Can you work these out from the drawing? Everything is in mm from the part's minimum corner. Coordinates: 2 decimals unless noted, no trailing zeros. Loops run counter-clockwise (first coordinate to the right, second up) from the corner with the lowest first, then second, coordinate; pieces in that order, holes last. Notation, with made-up numbers: (11, 87.25) - (32, 87.25) arc R21 ccw to (32, 102.25) - close; hole circle Ø10 at (51.5, 36). An arc over 180 degrees is marked (long way). Use CSV: the item, a comma, the result in double quotes.
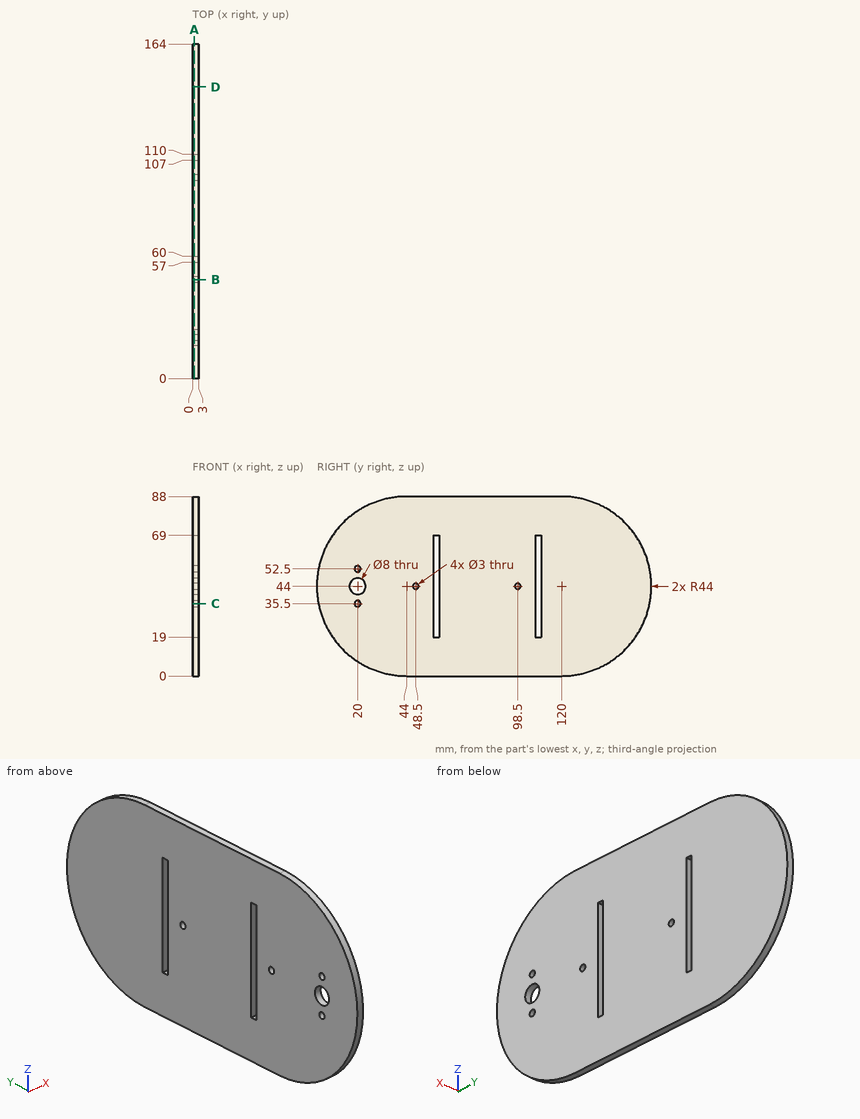
(1) Suppose I cut it at A-A (x = 0.8). Write out the boundary of the cut face in (y, z).
Computed:
outline,"(44, 0) - (120, 0) arc R44 ccw to (120, 88) - (44, 88) arc R44 ccw to start; hole circle Ø8 at (20, 44); hole circle Ø3 at (20, 35.5); hole circle Ø3 at (20, 52.5); hole circle Ø3 at (48.5, 44); hole (57, 19) - (60, 19) - (60, 69) - (57, 69) - close; hole circle Ø3 at (98.5, 44); hole (107, 19) - (110, 19) - (110, 69) - (107, 69) - close"
(2) Suppose I cut it at D-D (y = 143). Write out the boundary of the cut face in (x, z), plus the area to 3 significant figures.
Computed:
outline,"(0, 6.49) - (3, 6.49) - (3, 81.51) - (0, 81.51) - close"
area,"225 mm²"
(3) Please list where these lines run through material, in increasing order: line 1 (Y direction, x = 1.9, z = 44); line 2 (Y direction, x = 0.7, z = 67); line 3 (Y direction, x = 0.6, z = 35.5).
Computed:
line 1,"y = 0 to 16, 24 to 47, 50 to 57, 60 to 97, 100 to 107, 110 to 164"
line 2,"y = 6.49 to 57, 60 to 107, 110 to 157.51"
line 3,"y = 0.83 to 18.5, 21.5 to 57, 60 to 107, 110 to 163.17"
(4) Suppose I cut it at C-C (z = 35.5). Write out the boundary of the cut face in (x, y), plus the area to 3 significant figures.
Computed:
outline,"(0, 0.83) - (3, 0.83) - (3, 18.5) - (0, 18.5) - close; (0, 21.5) - (3, 21.5) - (3, 57) - (0, 57) - close; (0, 60) - (3, 60) - (3, 107) - (0, 107) - close; (0, 110) - (3, 110) - (3, 163.17) - (0, 163.17) - close"
area,"460 mm²"
(5) Will these pins go through, and if not, where does the flat tip stop? pin 1 (4 mm diameter, centred on y = 38.5, z = 35, fed in from -X); pin 2 (2.5 mm diameter, centred on y = 98.5, z = 44, fed in from -X); pin 3 (0.9 mm diameter, centred on x = 1.5, z = 53.5, fed in from -Y); pin 4 (1.5 mm diameter, centred on x = 0.5, z = 9, fed in from +Y).
Computed:
pin 1,"stops at x = 0"
pin 2,"passes through"
pin 3,"stops at y = 0.94"
pin 4,"stops at y = 147.62"
(6) Suppose I cut it at B-B (y = 48.5). Write out the boundary of the cut face in (x, z).
Computed:
outline,"(0, 0) - (3, 0) - (3, 42.5) - (0, 42.5) - close; (0, 45.5) - (3, 45.5) - (3, 88) - (0, 88) - close"
